```python
from build123d import *

# Parameters (mm, degrees)
F0_W        = 106.68
F0_H        = 106.68
F0_W_2      = 101.6
F0_H_2      = 101.6
F0_R        = 38.1
F1_DEPTH    = 8.89
F2_DEPTH    = 5.08
F3_DEPTH    = 7.366
F2_FACE_W   = 106.68
F2_FACE_H   = 106.68
F2_FACE_W_2 = 101.6
F2_FACE_H_2 = 101.6
F4_DEPTH    = 25.4


with BuildPart() as f1:
    # F0 (on Top) → F1 (new body)
    with BuildSketch(Plane.XY):
        Rectangle(F0_W, F0_H)
        Rectangle(F0_W_2, F0_H_2, mode=Mode.SUBTRACT)
        Rectangle(F0_W_2, F0_H_2)
        Circle(F0_R, mode=Mode.SUBTRACT)
        Circle(F0_R)
    extrude(amount=-F1_DEPTH)

    # F0 (on Top) → F2 (cut)
    with BuildSketch(Plane.XY):
        Rectangle(F0_W_2, F0_H_2)
        Circle(F0_R, mode=Mode.SUBTRACT)
    extrude(amount=-F2_DEPTH, mode=Mode.SUBTRACT)

    # F0 (on Top) → F3 (cut)
    with BuildSketch(Plane.XY):
        Circle(F0_R)
    extrude(amount=-F3_DEPTH, mode=Mode.SUBTRACT)

    # F2_face (on face) → F4 (join)
    with BuildSketch(Plane.XY):
        Rectangle(F2_FACE_W, F2_FACE_H)
        Rectangle(F2_FACE_W_2, F2_FACE_H_2, mode=Mode.SUBTRACT)
    extrude(amount=F4_DEPTH)


solid = f1.part
```
Check sheet for the modelled part. Datum: model origin and axes. Units: mm. A direction names the side the tool comes from. Round coordinates to 2 decimals unless told otherwise and drop trailing zeros. Loops run counter-clockwise (first coordinate to the right, second up) from the corner with the lowest first, then second, coordinate; pieces in that order, holes last. Notation, with made-up numbers: M 68,65.5 L 101,65.5 A21 ccw 101,75.5 Z; hole C 79.25,41.5 d8. An arc over 180 degrees is marked long. Answer as a JSON object with one key per item and string values.
1. Access from +Z, -Z, +X, -X, +Y, -Y to the whole of each face (thin tool, end or side, straight path). Record for faces 1 (the flat face through (53.34, -1, 8)), 2 (the flat face through (22, 35, -5.08)).
Reply:
{"face 1": "+Z, -Z, +X, +Y, -Y", "face 2": "+Z"}
2. Section check B-B (x = 0). Record the boundary of the cut face in (y, z).
Reply:
{"outline": "M -53.34,-8.89 L 53.34,-8.89 L 53.34,25.4 L 50.8,25.4 L 50.8,-5.08 L 38.1,-5.08 L 38.1,-7.37 L -38.1,-7.37 L -38.1,-5.08 L -50.8,-5.08 L -50.8,25.4 L -53.34,25.4 Z"}
3. Section check A-A (z = 4). Record the boundary of the cut face in (x, y).
Reply:
{"outline": "M -53.34,-53.34 L 53.34,-53.34 L 53.34,53.34 L -53.34,53.34 Z; hole M -50.8,-50.8 L 50.8,-50.8 L 50.8,50.8 L -50.8,50.8 Z"}
4. Scan lines: line 1 (X direction, y = 5, z = 21.5); line 2 (Y direction, x = 0, z = -6.2). Record each from-to range of solid material in increasing order.
Reply:
{"line 1": "x = -53.34 to -50.8, 50.8 to 53.34", "line 2": "y = -53.34 to -38.1, 38.1 to 53.34"}
5. Gauge pin test, flat end, axial feed: P1, Ø6, axis at x = -2, y = -39.5, coming from the +Z side. Record the tip position at first contact, or that the pin passes through.
Reply:
{"P1": "stops at z = -5.08"}
